from build123d import *

# Parameters (mm, degrees)
F0_W     = 80
F0_H     = 5.1
F0_W_2   = 20
F0_H_2   = 5
F1_DEPTH = 5
F2_W     = 20
F2_H     = 5
F2_W_2   = 40
F3_DEPTH = 7.5
F4_DEPTH = 22.4
F5_W     = 4.5
F5_H     = 5
F6_DEPTH = 9.5
F7_W     = 4.5
F7_H     = 5
F8_DEPTH = 9.5
F9_DEPTH = 7.5


with BuildPart() as f1:
    # F0 (on Front) → F1 (new body)
    with BuildSketch(Plane.XZ):
        Polygon((-54.556705, 45), (-54.556705, 0), (85.443295, 0), (85.443295, 45), (65.443295, 45), (65.443295, 40), (45.443295, 40), (45.443295, 45), (5.443295, 45), (5.443295, 40), (-14.556705, 40), (-14.556705, 45), align=None)
        with Locations((-4.556705, 7.55)):
            Rectangle(F0_W, F0_H, mode=Mode.SUBTRACT)
        with Locations((-4.556705, 32.5)):
            Rectangle(F0_W_2, F0_H_2, mode=Mode.SUBTRACT)
        with Locations((55.443295, 32.5)):
            Rectangle(F0_W_2, F0_H_2, mode=Mode.SUBTRACT)
        with Locations((55.443295, 42.5)):
            Rectangle(F0_W_2, F0_H_2)
        with Locations((-4.556705, 42.5)):
            Rectangle(F0_W_2, F0_H_2)
    extrude(amount=F1_DEPTH)

    # F2 (on face) → F3 (join)
    with BuildSketch(Plane(origin=(0, 0, 0), x_dir=(-1, 0, 0), z_dir=(0, 1, 0))):
        with Locations((-75.443295, 42.5)):
            Rectangle(F2_W, F2_H)
        with Locations((-25.443295, 42.5)):
            Rectangle(F2_W_2, F2_H)
        with Locations((34.556705, 42.5)):
            Rectangle(F2_W_2, F2_H)
    extrude(amount=F3_DEPTH)

    # F2 (on face) → F4 (join)
    with BuildSketch(Plane(origin=(0, 0, 0), x_dir=(-1, 0, 0), z_dir=(0, 1, 0))):
        with Locations((-55.443295, 42.5)):
            Rectangle(F2_W, F2_H)
        with Locations((4.556705, 42.5)):
            Rectangle(F2_W, F2_H)
    extrude(amount=F4_DEPTH)

    # F5 (on face) → F6 (join)
    with BuildSketch(Plane(origin=(0, 22.4, 0), x_dir=(-1, 0, 0), z_dir=(0, 1, 0))):
        with Locations((-67.693295, 42.5)):
            Rectangle(F5_W, F5_H)
        with Locations((-43.193295, 42.5)):
            Rectangle(F5_W, F5_H)
    extrude(amount=-F6_DEPTH)

    # F7 (on face) → F8 (join)
    with BuildSketch(Plane(origin=(0, 22.4, 0), x_dir=(-1, 0, 0), z_dir=(0, 1, 0))):
        with Locations((-7.693295, 42.5)):
            Rectangle(F7_W, F7_H)
        with Locations((16.806705, 42.5)):
            Rectangle(F7_W, F7_H)
    extrude(amount=-F8_DEPTH)

    # F2 (on face) → F9 (join)
    with BuildSketch(Plane(origin=(0, 0, 0), x_dir=(-1, 0, 0), z_dir=(0, 1, 0))):
        Polygon((14.556705, 40), (-5.443295, 40), (-45.443295, 40), (-65.443295, 40), (-85.443295, 40), (-85.443295, 35), (-65.443295, 35), (-45.443295, 35), (-5.443295, 35), (14.556705, 35), (54.556705, 35), (54.556705, 40), align=None)
    extrude(amount=F9_DEPTH)


solid = f1.part
CAD build for the part. Positions are in the model's coordinates, mm. A direction names the side the tool comes from. Round coordinates to 2 decimals unless told otherwise and drop trailing zeros. Loops run counter-clockwise (first coordinate to the right, second up) from the corner with the lowest first, then second, coordinate; pieces in that order, holes last.
(1) Cut at D-D (y = -1.25). Give the cut face in (x, z), plus the area to 3 significant figures.
(2) Drop flat-ended pins along their axis: pin 1 (12 mm diameter, centred on x = 55.5, y = 18.5, fed in from -Z); pin 2 (1.5 mm diameter, centred on y = 11.5, z = 42, fed in from -X); pin 3 (6 mm diameter, centred on x = -34, y = 9, fed in from -Z). Give the stop position or say it passes through.
(3) Cut at A-A (y = 17). Give the cut face in (x, z).
(4) Wall check: line 1 along Z through (x, y) = (55, -1.25); line 2 along X through (y, z) = (9.75, 43); line 3 along Z through (x, y) = (-19, -1). Give the ranges that are in metal, low to high.
(5) Cut at C-C (z = 32.5). Give the cut face in (x, y), plus the area to 3 significant figures.
(6) Which spindle directions (+Z, -Z, +X, -X, +Y, -Y) get a long thin tool onto all of the face, cutting with end or side? Do faces 3 (the flat face through (65.443, -2, 32)), 4 (the flat face through (43, 12.9, 43)), 5 (the flat face through (40.943, 18, 42)). Say none if no direction does.
(7) Cut at B-B (x = 49). Give the cut face in (y, z).
(8) Two-plate mould, pull along Z, no slides. Class faces 1 (the flat face through (5.443, -2, 32)), 2 (the flat face through (-14.557, 10, 42)): +Z half, -Z half, draft (parallel to the pull), parting line (faces both ways), or undercut.
Findings below:
1. outline: (-54.56, 0) - (85.44, 0) - (85.44, 45) - (-54.56, 45) - close; hole (-44.56, 5) - (35.44, 5) - (35.44, 10.1) - (-44.56, 10.1) - close; hole (-14.56, 30) - (5.44, 30) - (5.44, 35) - (-14.56, 35) - close; hole (45.44, 30) - (65.44, 30) - (65.44, 35) - (45.44, 35) - close
1. area: 5,690 mm2
2. pin 1: stops at z = 40
2. pin 2: stops at x = -14.56
2. pin 3: stops at z = 35
3. outline: (-19.06, 40) - (9.94, 40) - (9.94, 45) - (-19.06, 45) - close; (40.94, 40) - (69.94, 40) - (69.94, 45) - (40.94, 45) - close
4. line 1: z = 0 to 30, 35 to 45
4. line 2: x = -14.56 to 5.44, 45.44 to 65.44
4. line 3: z = 0 to 5, 10.1 to 45
5. outline: (-54.56, -5) - (-14.56, -5) - (-14.56, 0) - (-54.56, 0) - close; (5.44, -5) - (45.44, -5) - (45.44, 0) - (5.44, 0) - close; (65.44, -5) - (85.44, -5) - (85.44, 0) - (65.44, 0) - close
5. area: 500 mm2
6. face 3: +Y, -Y
6. face 4: +Z, -Z
6. face 5: +Z, -Z, +Y
7. outline: (-5, 0) - (0, 0) - (0, 30) - (-5, 30) - close; (-5, 35) - (7.5, 35) - (7.5, 40) - (22.4, 40) - (22.4, 45) - (-5, 45) - close
8. face 1: undercut
8. face 2: draft
